For this review, use the dimensioned drawing (mm, ordinates from the lowest corner) and the shaded views. A direction names the side the tool comes from. Coordinates: 2 decimals unless noted, no trailing zeros. Write each loop counter-clockwise with the first axis right and the second up, starting at its lowest first coordinate (ties: lowest second). Pieces come first, ordered by that corner, then holes.
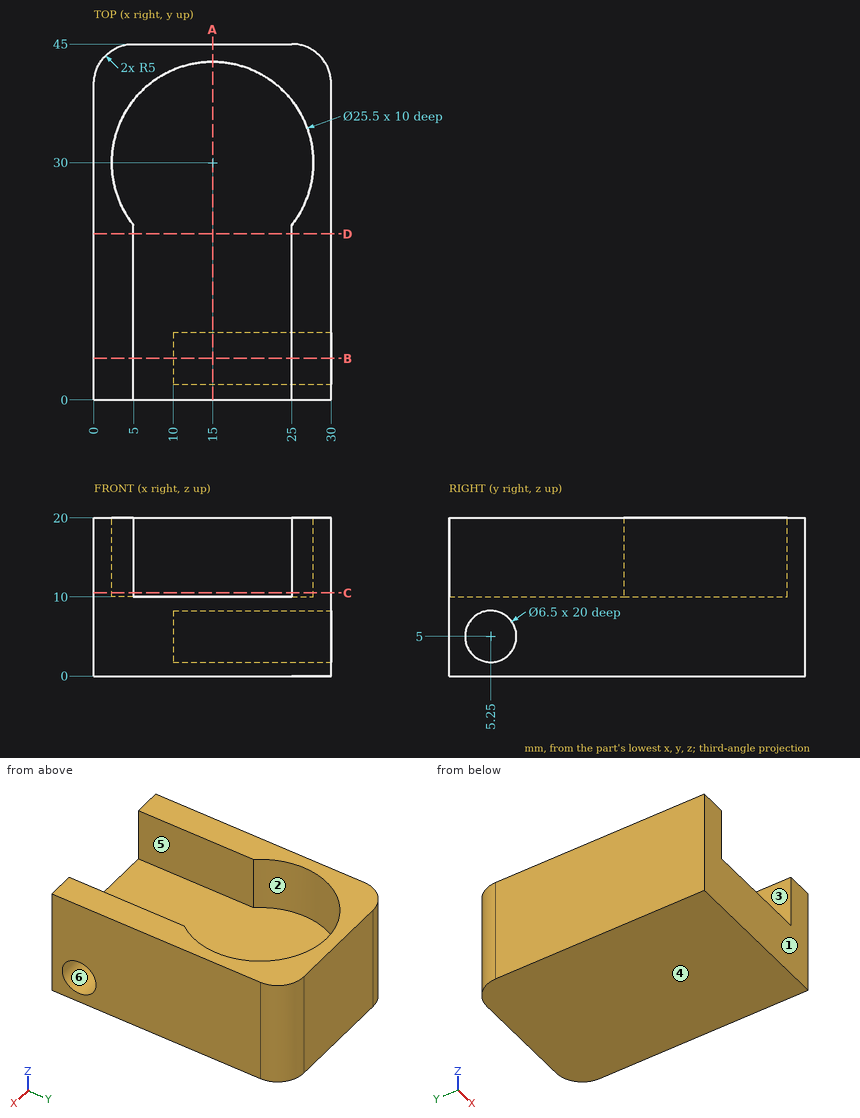
Item 1: Mouldability with a two-part tool opening along Z and no side actions: class the marked faces 4, 5 and 6 as pulls with the +Z half, pulls with the -Z half, needs draft (parallel to the pull), parting line crosses it, or undercut.
Solved:
face 4: pulls with the -Z half
face 5: needs draft
face 6: undercut
Item 2: Take a section at A-A, the plane x = 15. Write out the cut boundary in (y, z), plus the area to 3 significant figures.
Solved:
outline: (0, 0) - (45, 0) - (45, 20) - (42.75, 20) - (42.75, 10) - (0, 10) - close; hole circle Ø6.5 at (5.25, 5)
area: 439 mm2
Item 3: Machinability: for the marked faces 1, 2 and 3, which of the approach directions +Z, -Z, +X, -X, +Y, -Y give a long, thin tool a straight path to every point of the face, cutting with its end or side? Answer none if there is none.
Solved:
face 1: +Z, -Z, +X, -X, -Y
face 2: +Z
face 3: +Z, -Y
Item 4: Take a section at D-D, the plane y = 21. Write out the cut boundary in (x, z).
Solved:
outline: (0, 0) - (30, 0) - (30, 20) - (25, 20) - (25, 10) - (5, 10) - (5, 20) - (0, 20) - close
Item 5: To check wall thickness, follow line 1 along Z through (x, y) = (24, 5.25); line 2 along X through (y, z) = (19.5, 12.5); line 3 along Y through (x, z) = (15, 17.75). State the ranges of each line that lie inside material, in increasing order.
Solved:
line 1: z = 0 to 1.75, 8.25 to 10
line 2: x = 0 to 5, 25 to 30
line 3: y = 42.75 to 45
Item 6: For pin 1 (4 mm diameter, centred on y = 5.25, z = 5, fed in from +X), flat-tipped, find the tip position at first contact; note if it passes through.
Solved:
pin 1: stops at x = 10
Item 7: Take a section at B-B, the plane y = 5.25. Write out the cut boundary in (x, z).
Solved:
outline: (0, 0) - (30, 0) - (30, 1.75) - (10, 1.75) - (10, 8.25) - (30, 8.25) - (30, 20) - (25, 20) - (25, 10) - (5, 10) - (5, 20) - (0, 20) - close
Item 8: Take a section at C-C, the plane z = 10.5. Write out the cut boundary in (x, y), plus the area to 3 significant figures.
Solved:
outline: (0, 0) - (5, 0) - (5, 22.09) arc R12.75 cw (long way) to (25, 22.09) - (25, 0) - (30, 0) - (30, 40) arc R5 ccw to (25, 45) - (5, 45) arc R5 ccw to (0, 40) - close
area: 454 mm2
